```python
from build123d import *

# Parameters (mm, degrees)
SKETCH1_R           = 2.032
BOSS_EXTRUDE1_DEPTH = 3.0861


with BuildPart() as part:
    # Sketch1 → Boss-Extrude1 (new body)
    with BuildSketch(Plane(origin=(0, 0, 0), x_dir=(1, 0, 0), z_dir=(0, 1, 0))):
        with BuildLine():
            Line((-2.6924, 4.4704), (28.98404818, 4.4704))
            ThreePointArc((28.98404818, 4.4704), (29.793051754, 4.179385811), (30.23129703, 3.439712155))
            Line((30.23129703, 3.439712155), (35.572400198, -24.397088649))
            ThreePointArc((35.572400198, -24.397088649), (35.589450767, -24.516205211), (35.595151349, -24.636400804))
            Line((35.595151349, -24.636400804), (35.595151349, -40.835711832))
            ThreePointArc((35.595151349, -40.835711832), (35.223176961, -41.733737444), (34.325151349, -42.105711832))
            Line((34.325151349, -42.105711832), (2.465757874, -42.105711832))
            ThreePointArc((2.465757874, -42.105711832), (1.800944431, -41.917803827), (1.332861331, -41.409685196))
            Line((1.332861331, -41.409685196), (-3.825296543, -31.228621763))
            ThreePointArc((-3.825296543, -31.228621763), (-3.927648681, -30.949708893), (-3.9624, -30.6546484))
            Line((-3.9624, -30.6546484), (-3.9624, 3.2004))
            ThreePointArc((-3.9624, 3.2004), (-3.590425612, 4.098425612), (-2.6924, 4.4704))
        make_face()
        with Locations(Location((0, 0, 0), (0, 0, 270))):
            Circle(SKETCH1_R, mode=Mode.SUBTRACT)
        with Locations(Location((26.3652, 0, 0), (0, 0, 270))):
            Circle(SKETCH1_R, mode=Mode.SUBTRACT)
        with Locations(Location((5.242151349, -37.660711832, 0), (0, 0, 270))):
            Circle(SKETCH1_R, mode=Mode.SUBTRACT)
        with Locations(Location((31.607351349, -37.660711832, 0), (0, 0, 270))):
            Circle(SKETCH1_R, mode=Mode.SUBTRACT)
        with BuildLine():
            Line((12.5603, 1.4859), (18.0213, 1.4859))
            ThreePointArc((18.0213, 1.4859), (19.817351224, 0.741951224), (20.5613, -1.0541))
            Line((20.5613, -1.0541), (20.5613, -4.374589338))
            ThreePointArc((20.5613, -4.374589338), (21.042661976, -5.86240972), (22.304299596, -6.786308716))
            Line((22.304299596, -6.786308716), (23.138687105, -7.062048584))
            ThreePointArc((23.138687105, -7.062048584), (24.000408807, -7.550166917), (24.609958316, -8.330726456))
            Line((24.609958316, -8.330726456), (33.329522963, -25.633983509))
            ThreePointArc((33.329522963, -25.633983509), (33.532385694, -26.189577102), (33.601251349, -26.777025014))
            Line((33.601251349, -26.777025014), (33.601251349, -28.923111832))
            ThreePointArc((33.601251349, -28.923111832), (32.857302573, -30.719163056), (31.061251349, -31.463111832))
            Line((31.061251349, -31.463111832), (24.165151349, -31.463111832))
            ThreePointArc((24.165151349, -31.463111832), (22.369100125, -32.207060608), (21.625151349, -34.003111832))
            Line((21.625151349, -34.003111832), (21.625151349, -36.581211832))
            ThreePointArc((21.625151349, -36.581211832), (20.881202573, -38.377263056), (19.085151349, -39.121211832))
            Line((19.085151349, -39.121211832), (13.649551349, -39.121211832))
            ThreePointArc((13.649551349, -39.121211832), (11.853500125, -38.377263056), (11.109551349, -36.581211832))
            Line((11.109551349, -36.581211832), (11.109551349, -34.003111832))
            ThreePointArc((11.109551349, -34.003111832), (10.365602573, -32.207060608), (8.569551349, -31.463111832))
            Line((8.569551349, -31.463111832), (0.5588, -31.463111832))
            ThreePointArc((0.5588, -31.463111832), (-1.237251224, -30.719163056), (-1.9812, -28.923111832))
            Line((-1.9812, -28.923111832), (-1.9812, -26.531672272))
            ThreePointArc((-1.9812, -26.531672272), (-1.956276805, -26.176723455), (-1.881996329, -25.828740353))
            Line((-1.881996329, -25.828740353), (3.23891195, -8.047368081))
            ThreePointArc((3.23891195, -8.047368081), (4.15226713, -6.72088542), (5.679708279, -6.2103))
            Line((5.679708279, -6.2103), (7.4803, -6.2103))
            ThreePointArc((7.4803, -6.2103), (9.276351224, -5.466351224), (10.0203, -3.6703))
            Line((10.0203, -3.6703), (10.0203, -1.0541))
            ThreePointArc((10.0203, -1.0541), (10.764248776, 0.741951224), (12.5603, 1.4859))
        make_face(mode=Mode.SUBTRACT)
    extrude(amount=BOSS_EXTRUDE1_DEPTH)


solid = part.part
```
Here's how the part is built. I have some questions about the finished solid (model axes, mm). A direction names the side the tool comes from. Round coordinates to 2 decimals unless told otherwise and drop trailing zeros. Loops run counter-clockwise (first coordinate to the right, second up) from the corner with the lowest first, then second, coordinate; pieces in that order, holes last. Notation, with made-up numbers: (64.5, -16.75) -> (88.5, -16.75) arc R14 ccw to (88.5, 6.25) -> close; hole circle Ø7 at (-28, -34.75). An arc over 180 degrees is marked (long way). Answer as CSV lines item,"result". Start each with the question number.
1. I need wall thicknesses on probe 1 along X at (y, z) = (2.5, 27); probe 2 along Z at (x, y) = (27.5, 0.6); probe 3 along X at (y, z) = (1.4, 0). Which ranges of each line are inside material? Lowest first, please. Write a range as from..to.
2. Imagine slicing it at B-B on z = 38. Write out the boundary of the cut face in (x, y), plus the area to 3 significant figures.
3. Imagine slicing it at C-C on x = 0. Write out the boundary of the cut face in (y, z), plus the area to 3 significant figures.
4. Imagine slicing it at A-A on x = 15. Write out the boundary of the cut face in (y, z), plus the area to 3 significant figures.
5. Imagine slicing it at D-D on y = 2.4. State how many separate pieces and enclosed holes the cut face has, plus the area to 3 significant figures.
6. For faces 5 (the face through (32.877, 1.521, 30.699)), 6 (the face through (-1.21, 1.52, 36.39)), which set-ups out of +Z, -Z, +X, -X, +Y, -Y let a thin tool reach every point of the face, with its end or its side?
7. If we mould it in two halves opening along X, with no side actions, what happens to faces 1 (the face through (9.256, 1.521, 5.486)), 2 (the face through (5.85, 1.52, 39.6)), 3 (the face through (25, 0, 8)), 4 (the face through (-3.962, 2, 14))? For each: pulls with the +X half, pulls with the -X half, needs draft (parallel to the pull), parting line crosses it, or undercut.
8. I'm going to push a flat-ended pin straight in: P1, Ø1.3, axis at y = 1.5, z = 2, coming from the +X side. Where does the tip first touch, or does it pass through?
Solution:
1,probe 1,"-3.96..-1.98, 33.6..35.6"
1,probe 2,"-4.47..-1.69, 1.69..14.07, 31.46..42.11"
1,probe 3,"-3.96..-2.03, 2.03..10.25, 20.33..24.33, 28.4..30.89"
2,outline,"(-0.39, 0) -> (3.24, 0) -> (3.24, 3.09) -> (-0.39, 3.09) -> close; (7.25, 0) -> (11.54, 0) -> (11.54, 3.09) -> (7.25, 3.09) -> close; (21.19, 0) -> (29.6, 0) -> (29.6, 3.09) -> (21.19, 3.09) -> close; (33.61, 0) -> (35.6, 0) -> (35.6, 3.09) -> (33.61, 3.09) -> close"
2,area,"56.6 mm²"
3,outline,"(0, -4.47) -> (3.09, -4.47) -> (3.09, -2.03) -> (0, -2.03) -> close; (0, 2.03) -> (3.09, 2.03) -> (3.09, 19.29) -> (0, 19.29) -> close; (0, 31.4) -> (3.09, 31.4) -> (3.09, 38.78) -> (0, 38.78) -> close"
3,area,"83.6 mm²"
4,outline,"(0, -4.47) -> (3.09, -4.47) -> (3.09, -1.49) -> (0, -1.49) -> close; (0, 39.12) -> (3.09, 39.12) -> (3.09, 42.11) -> (0, 42.11) -> close"
4,area,"18.4 mm²"
5,separate pieces,"1"
5,enclosed holes,"5"
5,area,"781 mm²"
6,face 5,"+Y, -Y"
6,face 6,"+Z, -X, +Y, -Y"
7,face 1,"undercut"
7,face 2,"undercut"
7,face 3,"needs draft"
7,face 4,"pulls with the -X half"
8,P1,"x = 31.4"
